```python
from build123d import *

# Parameters (mm, degrees)
F0_W        = 10
F0_H        = 8
F1_DEPTH    = 15
F2_R        = 4
F2_R_2      = 3
F3_DEPTH    = 25
F4_DEPTH    = 5
F5_SIZE     = 0.99999
F6_SIZE     = 2
F7_T1_DEPTH = 15
F7_T3_DEPTH = 19.9705627485
F7_T5_DEPTH = 16.7612260356
F8_R        = 1


# Not quite as in the source:
# - a fillet or chamfer that OpenCascade refuses, or shapes differently, is made with other operations: its cross-section is extruded or revolved along the edge and cut away or added
# - a fillet or chamfer is up to 0.001 mm smaller than in the source, because OpenCascade refuses the exact size


with BuildPart() as f1:
    # F0 (on Top) → F1 (new body)
    with BuildSketch(Plane.XY):
        Polygon((20, -8), (0, -8), (0, 0), (-5, 0), (-5, -11), (20, -11), align=None)
        with Locations((25, -4)):
            Rectangle(F0_W, F0_H)
        Polygon((30, -8), (20, -8), (20, -11), align=None)
    extrude(amount=F1_DEPTH)

    # F2 (on face) → F3 (cut)
    with BuildSketch(Plane(origin=(0, 0, 0), x_dir=(-1, 0, 0), z_dir=(0, 1, 0))):
        with Locations((-25, 7.5)):
            Circle(F2_R)
        with Locations((-25, 7.5)):
            Circle(F2_R_2, mode=Mode.SUBTRACT)
        with Locations((-25, 7.5)):
            Circle(F2_R_2)
    extrude(amount=-F3_DEPTH, mode=Mode.SUBTRACT)

    # F2 (on face) → F4 (join)
    with BuildSketch(Plane(origin=(0, 0, 0), x_dir=(-1, 0, 0), z_dir=(0, 1, 0))):
        with Locations((-25, 7.5)):
            Circle(F2_R)
        with Locations((-25, 7.5)):
            Circle(F2_R_2, mode=Mode.SUBTRACT)
    extrude(amount=-F4_DEPTH)

    # F5 (size 1 in the source; OpenCascade refuses exactly that, so slightly less here)
    f5_edges = [f1.edges().sort_by_distance(p)[0] for p in [
        (28, -5, 7.5),
    ]]
    chamfer(f5_edges, length=F5_SIZE)

    # F6
    f6_edges = [f1.edges().sort_by_distance(p)[0] for p in [
        (-5, 0, 7.5),
        (0, 0, 7.5),
        (-5, -11, 7.5),
    ]]
    chamfer(f6_edges, length=F6_SIZE)

    # F7: fillet of radius 2.4 on 8 edges, made by hand

    # F7_s2 → F7_t1 (join)
    with BuildSketch(Plane.XY):
        with BuildLine():
            ThreePointArc((0, -5.6), (0.7029437252, -7.2970562748), (2.4, -8))
            Line((2.4, -8), (0, -8))
            Line((0, -8), (0, -5.6))
        make_face()
        with BuildLine():
            ThreePointArc((17.6, -8), (19.2970562748, -7.2970562748), (20, -5.6))
            Line((20, -5.6), (20, -8))
            Line((20, -8), (17.6, -8))
        make_face()
    extrude(amount=F7_T1_DEPTH)

    # F7_s4 → F7_t3 (cut)
    with BuildSketch(Plane.XY.offset(-2.4852813742)):
        with BuildLine():
            ThreePointArc((-1.2970562748, -0.7029437252), (-2.075672312, -0.182689122), (-2.9941125497, 0))
            Line((-2.9941125497, 0), (-2, 0))
            Line((-2, 0), (-1.2970562748, -0.7029437252))
        make_face()
        with BuildLine():
            ThreePointArc((-2.0058874503, 0), (-2.924327688, -0.182689122), (-3.7029437252, -0.7029437252))
            Line((-3.7029437252, -0.7029437252), (-3, 0))
            Line((-3, 0), (-2.0058874503, 0))
        make_face()
        with BuildLine():
            ThreePointArc((-4.2970562748, -1.2970562748), (-4.817310878, -2.075672312), (-5, -2.9941125497))
            Line((-5, -2.9941125497), (-5, -2))
            Line((-5, -2), (-4.2970562748, -1.2970562748))
        make_face()
        with BuildLine():
            ThreePointArc((-5, -8.0058874503), (-4.817310878, -8.924327688), (-4.2970562748, -9.7029437252))
            Line((-4.2970562748, -9.7029437252), (-5, -9))
            Line((-5, -9), (-5, -8.0058874503))
        make_face()
        with BuildLine():
            ThreePointArc((-3.7029437252, -10.2970562748), (-2.924327688, -10.817310878), (-2.0058874503, -11))
            Line((-2.0058874503, -11), (-3, -11))
            Line((-3, -11), (-3.7029437252, -10.2970562748))
        make_face()
    extrude(amount=F7_T3_DEPTH, mode=Mode.SUBTRACT)

    # F7_s6 → F7_t5 (cut)
    with BuildSketch(Plane.XY.offset(-0.8806130178)):
        with BuildLine():
            ThreePointArc((20.3373897182, -10.8987830845), (19.9962663401, -10.9745609492), (19.6477547929, -11))
            Line((19.6477547929, -11), (20, -11))
            Line((20, -11), (20.3373897182, -10.8987830845))
        make_face()
    extrude(amount=F7_T5_DEPTH, mode=Mode.SUBTRACT)

    # F8
    f8_edges = [f1.edges().sort_by_distance(p)[0] for p in [
        (-2.5, -0.051415, 7.5),
        (0, -2, 7.5),
        (30, -8, 7.5),
    ]]
    fillet(f8_edges, radius=F8_R)


solid = f1.part
```
The model under review builds one solid part; all positions refer to its coordinate system, in mm. A direction names the side the tool comes from. Round coordinates to 2 decimals unless told otherwise and drop trailing zeros. Write each loop counter-clockwise with the first axis right and the second up, starting at its lowest first coordinate (ties: lowest second). Pieces come first, ordered by that corner, then holes. Notation, with made-up numbers: (66.5, 25.5) - (88.5, 25.5) arc R12 cw to (88.5, 34.5) - close; hole circle Ø10 at (82.25, 74.5). An arc over 180 degrees is marked (long way). Use one line per item in the form item = value.
Q1. Consider section D-D (y = -9). State the section outline as (x, z) points.
Answer key:
outline = (-4.78, 0) - (26.67, 0) - (26.67, 3.86) arc R4 cw (long way) to (26.67, 11.14) - (26.67, 15) - (-4.78, 15) - close
Q2. Tool access review of faces 4 (the flat face through (28.4, 0, 7.6)), 5 (the flat face through (-1, -1, 7)): name each direction out of +Z, -Z, +X, -X, +Y, -Y from which nothing blocks a thin tool from reaching the whole face with its end or side.
Answer key:
face_4 = +Z, -Z, +X, -X, +Y
face_5 = +Z, -Z, +Y
Q3. Consider section C-C (y = -6.5). State the section outline as (x, z) points, and give its area (3 significant figures).
Answer key:
outline = (-5, 0) - (0.18, 0) - (0.18, 15) - (-5, 15) - close; (19.82, 0) - (30, 0) - (30, 15) - (19.82, 15) - close; hole circle Ø8 at (25, 7.5)
area = 180 mm2
Q4. Consider section A-A (y = -4.5). State the section outline as (x, z) points.
Answer key:
outline = (-5, 0) - (0, 0) - (0, 15) - (-5, 15) - close; (20, 0) - (30, 0) - (30, 15) - (20, 15) - close; hole circle Ø7 at (25, 7.5)
Q5. For line 1 (Z direction, x = 25, y = -2.15); line 2 (X direction, y = -3, z = 3.5); line 3 (Z direction, x = 25, y = -7.95), list the stretches that pass through material, from the lowest coordinate up. Write a range as [from, to].
Answer key:
line_1 = [0, 4.5], [10.5, 15]
line_2 = [-5, 0], [20, 30]
line_3 = [0, 3.5], [11.5, 15]
Q6. Draft analysis for pull direction X (two halves, no side actions). For faces 1 (the flat face through (20, -3, 7)), 2 (the flat face through (20.77, -10.77, 7.4)), 3 (the flat face through (-5, -5, 7)), state which applies: +X half, -X half, draft (parallel to the pull), parting line (faces both ways), or undercut.
Answer key:
face_1 = undercut
face_2 = +X half
face_3 = -X half
Q7. Insertion check: pin 1 Ø4 at (x, z) = (24.5, 9) entering from -Y; pin 2 Ø4.5 at (x, z) = (8.5, 6.5) entering from +Y; pin 3 Ø3 at (x, y) = (0.5, -3.5) entering from +Z; pin 4 Ø6.5 at (x, z) = (25, 7.5) entering from -Y. Each pin has a flat end and moves straight along its axis. Give the tip position at first contact, or say it passes through.
Answer key:
pin_1 = -4.58
pin_2 = -8
pin_3 = 15
pin_4 = -4.25
